Design review of the part built by this model. Coordinates are the model's own, in mm. Face numbers are marked on the shaded views. A direction names the side the tool comes from. Coordinates: 2 decimals unless noted, no trailing zeros. Write each loop counter-clockwise with the first axis right and the second up, starting at its lowest first coordinate (ties: lowest second). Pieces come first, ordered by that corner, then holes. Notation, with made-up numbers: (-4, 70.5) -> (16, 70.5) arc R27 cw to (16, 97.5) -> close; hole circle Ø1 at (-5.5, -25.75). An arc over 180 degrees is marked (long way). Return JSON: item names as keys, results as strings. Group by question number.
from build123d import *

# Parameters (mm, degrees)
F0_W            = 25
F0_H            = 40
F1_DEPTH        = 1.5
F4_W            = 25
F4_H            = 40
F5_DEPTH        = 1.5
F1_FACE_W       = 25
F1_FACE_H       = 3
F8_D            = 5
F8_CSINK_D      = 10
F8_CSINK_ANGLE  = 90
F10_D           = 5
F10_CSINK_D     = 10
F10_CSINK_ANGLE = 90


with BuildPart() as f1:
    # F0 (on Front) → F1 (new body, symmetric)
    with BuildSketch(Plane.XZ):
        with Locations((0, -20)):
            Rectangle(F0_W, F0_H)
    extrude(amount=F1_DEPTH, both=True)



with BuildPart() as f5:
    # F4 (on face) → F5 (new body, symmetric)
    with BuildSketch(Plane(origin=(0, 0, 0), x_dir=(-0.5, -0.866025, 0), z_dir=(-0.866025, 0.5, 0))):
        with Locations((0, 60)):
            Rectangle(F4_W, F4_H)
    extrude(amount=F5_DEPTH, both=True)


with BuildPart() as f1_1:
    add(f1.part)

    add(f5.part)  # F6 merges F5
    # F1_face (on face) → F6 section 0
    with BuildSketch(Plane.XY):
        Rectangle(F1_FACE_W, F1_FACE_H)
    # F5_face (on face) → F6 section 1
    with BuildSketch(Plane(origin=(0, 0, 40), x_dir=(1, 0, 0), z_dir=(0, 0, -1))):
        Polygon((7.549038, -10.075318), (-4.950962, 11.575318), (-7.549038, 10.075318), (4.950962, -11.575318), align=None)
    loft()

    # F8 (through all)
    with Locations(Plane(origin=(0, 1.5, 0), x_dir=(-1, 0, 0), z_dir=(0, 1, 0))):
        with Locations((0, -32), (0, -16)):
            CounterSinkHole(F8_D / 2, F8_CSINK_D / 2, counter_sink_angle=F8_CSINK_ANGLE)

    # F10 (through all)
    with Locations(Plane(origin=(1.299038, -0.75, 0), x_dir=(0.5, 0.866025, 0), z_dir=(0.866025, -0.5, 0))):
        with Locations((0, 72), (0, 52)):
            CounterSinkHole(F10_D / 2, F10_CSINK_D / 2, counter_sink_angle=F10_CSINK_ANGLE)


solid = f1_1.part
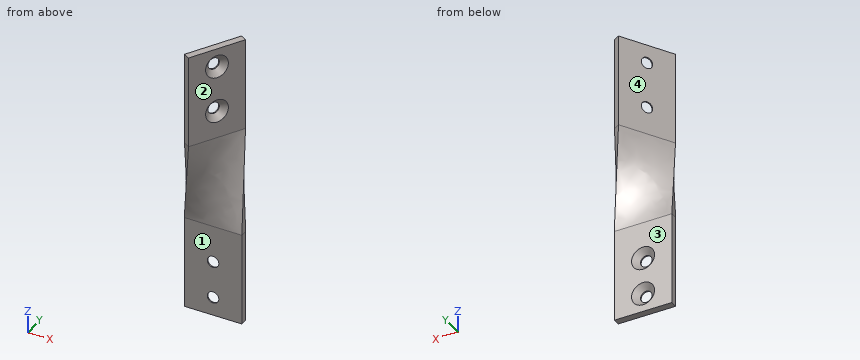
Q1. We need section B-B on z = 59.5. Write out the cut boundary in (x, y), plus the area to 3 significant figures.
Q2. We need section A-A on z = -16. Write out the cut boundary in (x, y).
Q3. Wall thickness on L1, parallel to X at y = -1.1, z = -32; L2, parallel to Z at x = 0, y = -1.3; L3, parallel to Y at x = 7, z = -23.5: over which ranges is each line inside the solid? List them lowest first.
Q4. For P1, Ø7.5, axis at x = 3.5, z = -25, coming from the +Y side; P2, Ø1, axis at y = 7, z = 61.5, coming from the +X side; P3, Ø6.5, axis at x = 0, z = -32, coming from the -Y side, all flat-tipped, find the tip position at first contact; note any pin that passes through.
Q5. For the marked faces 1, 2, 3 and 4, list the 3-axis set-ups (+Z, -Z, +X, -X, +Y, -Y) from which the entire face can be reached by the end or side of a thin tool; tool diameter is ignored.
Findings below:
{
 "1": {"outline": "(-7.55, -10.08) -> (-4.95, -11.58) -> (7.55, 10.08) -> (4.95, 11.58) -> close", "area": "75.0 mm^2"},
 "2": {"outline": "(-12.5, -1.5) -> (-2.5, -1.5) -> (-2.5, -1) -> (-5, 1.5) -> (-12.5, 1.5) -> close; (2.5, -1.5) -> (12.5, -1.5) -> (12.5, 1.5) -> (5, 1.5) -> (2.5, -1) -> close"},
 "3": {"L1": "x = -12.5 to -2.5, 2.5 to 12.5", "L2": "z = -40 to -34.5, -29.5 to -18.5, -13.5 to 48.01, 55.99 to 68.01, 75.99 to 80", "L3": "y = -1.5 to 1.5"},
 "4": {"P1": "stops at y = 1.5", "P2": "stops at x = 6.06", "P3": "stops at y = -1.5"},
 "5": {"face 1": "-Z, +X, -X, -Y", "face 2": "+Z, +X, -Y", "face 3": "-Z, +X, -X, +Y", "face 4": "+Z, -X, +Y"}
}
